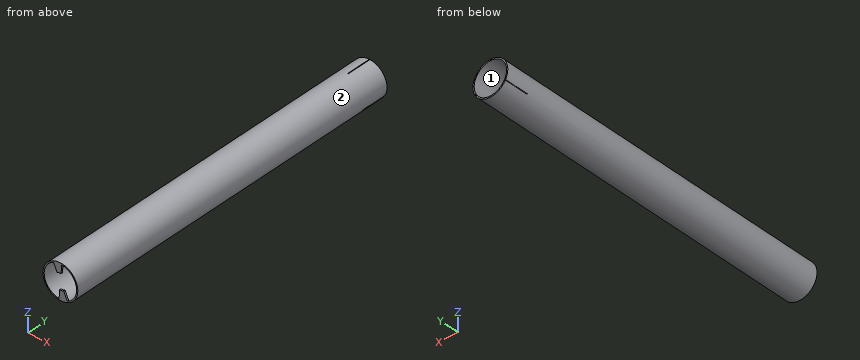
```python
from build123d import *

# Parameters (mm, degrees)
SKETCH1_R           = 57.5
BOSS_EXTRUDE1_DEPTH = 570
SHELL1_T            = -4
CUT_EXTRUDE4_DEPTH  = 80
CIRPATTERN1_COUNT   = 3
BOSS_EXTRUDE3_START = -5
BOSS_EXTRUDE3_DEPTH = 5


with BuildPart() as part:
    # Sketch1 → Boss-Extrude1 (new, symmetric)
    with BuildSketch(Plane(origin=(0, 0, 0), x_dir=(1, 0, 0), z_dir=(0, 1, 0))):
        with Locations(Location((0, 0, 0), (0, 0, 270))):
            Circle(SKETCH1_R)
    extrude(amount=BOSS_EXTRUDE1_DEPTH, both=True)

    # Shell1
    shell1_openings = [part.faces().sort_by_distance(p)[0] for p in [
        (0, 570, 0),
        (0, -570, 0),
    ]]
    offset(amount=SHELL1_T, openings=shell1_openings, kind=Kind.INTERSECTION)

    # Sketch2 → Cut-Extrude4 (cut)
    with BuildSketch(Plane(origin=(0, 570, 0), x_dir=(1, 0, 0), z_dir=(0, 1, 0))):
        with BuildLine():
            Line((1, -57.49130369), (1, -56.50869631))
            Line((1, -56.50869631), (4, -56.50869631))
            Line((4, -56.50869631), (4, -55.50869631))
            Line((4, -55.50869631), (0, -54.50869631))
            Line((0, -54.50869631), (-4, -55.50869631))
            Line((-4, -55.50869631), (-4, -56.50869631))
            Line((-4, -56.50869631), (-1, -56.50869631))
            Line((-1, -56.50869631), (-1, -57.49130369))
            ThreePointArc((-1, -57.49130369), (0, -57.5), (1, -57.49130369))
        make_face()
    cut_extrude4 = extrude(amount=-CUT_EXTRUDE4_DEPTH, mode=Mode.SUBTRACT)

    # CirPattern1: Cut-Extrude4 ×3 about axis
    cirpattern1_axis = Axis((0, 0, 0), (0, 1, 0))
    for i in range(1, CIRPATTERN1_COUNT):
        add(cut_extrude4.rotate(cirpattern1_axis, i * 360 / CIRPATTERN1_COUNT), mode=Mode.SUBTRACT)

    # Sketch4 → Boss-Extrude3 (add)
    with BuildSketch(Plane(origin=(0, -570, 0), x_dir=(-1, 0, 0), z_dir=(0, -1, 0)).offset(BOSS_EXTRUDE3_START)):
        with BuildLine():
            Line((4.482088094, 53.311920677), (2.136322363, 25.410354715))
            ThreePointArc((2.136322363, 25.410354715), (-4.5131548, 25.097438789), (-10.855067921, 23.074173884))
            Line((-10.855067921, 23.074173884), (-22.774358187, 48.410521678))
            ThreePointArc((-22.774358187, 48.410521678), (-9.468775757, 52.655410792), (4.482088094, 53.311920677))
        make_face()
        with BuildLine():
            Line((-4.482088094, -53.311920677), (-2.136322363, -25.410354715))
            ThreePointArc((-2.136322363, -25.410354715), (4.5131548, -25.097438789), (10.855067921, -23.074173884))
            Line((10.855067921, -23.074173884), (22.774358187, -48.410521678))
            ThreePointArc((22.774358187, -48.410521678), (9.468775757, -52.655410792), (-4.482088094, -53.311920677))
        make_face()
    extrude(amount=BOSS_EXTRUDE3_DEPTH)


solid = part.part
```
Geometry: final body of the model. Coordinates: model frame, mm. Face numbers are marked on the shaded views. Coordinates: 2 decimals unless noted, no trailing zeros. Order: outer loops, then holes, each group sorted by start corner. A loop starts at its lowest first (then second) coordinate and runs counter-clockwise, first axis right, second up.
Item 1: Section query B-B (x = -33.5). Output: boundary loops of the cut face in (y, z).
Answer:
outline: (-570, -46.73) - (570, -46.73) - (570, -41.71) - (-570, -41.71) - close; (-570, 41.71) - (570, 41.71) - (570, 46.73) - (-570, 46.73) - close
Item 2: Section query C-C (y = -225). Output: boundary loops of the cut face in (x, z), then the cut area to 3 significant figures.
Answer:
outline: circle Ø115 at (0, 0); hole circle Ø107 at (0, 0)
area: 1,390 mm2
Item 3: Draft query along X for the marked faces 1 and 2. Return one class per face: released by +X, released by -X, zero draft, split by the parting line, or undercut.
Answer:
face 1: undercut
face 2: split by the parting line
Item 4: Material intervals for line 1 along Z through (x, y) = (0, 325); line 2 along X through (y, z) = (-264, -5), sorted ascending.
Answer:
line 1: z = -57.5 to -53.5, 53.5 to 57.5
line 2: x = -57.28 to -53.27, 53.27 to 57.28
Item 5: Section query A-A (z = 0). Output: boundary loops of the cut face in (x, y), then the cut area to 3 significant figures.
Answer:
outline: (-57.5, -570) - (-53.5, -570) - (-53.5, 570) - (-57.5, 570) - close; (53.5, -570) - (57.5, -570) - (57.5, 570) - (53.5, 570) - close
area: 9,120 mm2
Item 6: Contact query for flat-ended pins moving along their axis: P1, Ø12, axis at x = -17, y = 374.5, coming from the +Z side; P2, Ø1.5, axis at x = 22.5, y = 340, coming from the -Z side; P3, Ø4, axis at x = -25.5, z = 42.5, coming from the -Y side; P4, Ø3, axis at y = -291.5, z = -15, coming from the +X side. Output: stop coordinate, or through.
Answer:
P1: stops at z = 56.44
P2: stops at z = -53.23
P3: passes through
P4: stops at x = 55.89
